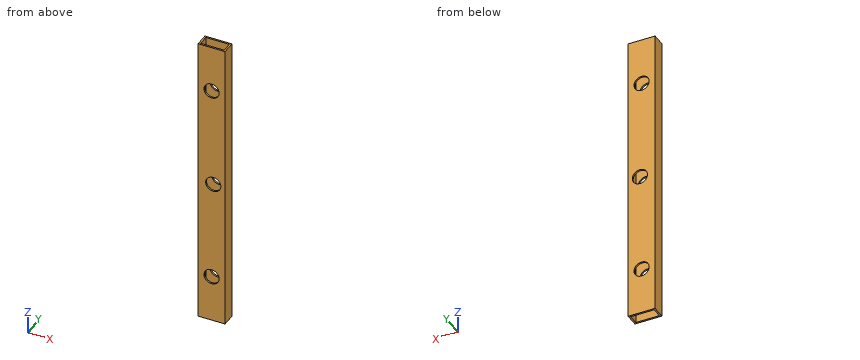
```python
from build123d import *

# Parameters (mm, degrees)
SKETCH1_W           = 50.8
SKETCH1_H           = 25.4
SKETCH1_W_2         = 44.45
SKETCH1_H_2         = 19.05
BOSS_EXTRUDE1_DEPTH = 558.8
SKETCH2_R           = 14.2875
CUT_EXTRUDE1_DEPTH  = 562.678947442


with BuildPart() as part:
    # Sketch1 → Boss-Extrude1 (new body)
    with BuildSketch(Plane.XY):
        with Locations((25.4, 12.7)):
            Rectangle(SKETCH1_W, SKETCH1_H)
        with Locations((25.4, 12.7)):
            Rectangle(SKETCH1_W_2, SKETCH1_H_2, mode=Mode.SUBTRACT)
    extrude(amount=BOSS_EXTRUDE1_DEPTH)

    # Sketch2 → Cut-Extrude1 (cut, through all)
    with BuildSketch(Plane(origin=(0, 25.4, 0), x_dir=(1, 0, 0), z_dir=(0, 1, 0))):
        with Locations(Location((28.575, -279.4, 0), (0, 0, 270))):
            Circle(SKETCH2_R)
        with Locations(Location((25.4, -469.9, 0), (0, 0, 270))):
            Circle(SKETCH2_R)
        with Locations(Location((25.4, -88.9, 0), (0, 0, 90))):
            Circle(SKETCH2_R)
    extrude(amount=-CUT_EXTRUDE1_DEPTH, mode=Mode.SUBTRACT)


solid = part.part
```
CAD build for the part. Positions are in the model's coordinates, mm. Round coordinates to 2 decimals unless told otherwise and drop trailing zeros. Order: outer loops, then holes, each group sorted by start corner. A loop starts at its lowest first (then second) coordinate and runs counter-clockwise, first axis right, second up. Notation, with made-up numbers: (16, 21.25) - (54, 21.25) arc R21 ccw to (54, 30.25) - close; hole circle Ø7 at (23.25, 60.25). An arc over 180 degrees is marked (long way). Answer in a Markdown table with one row per item. Add a question column.
(1) Band-saw the part on A-A on y = 11.5. List the corners of the cut face in (x, z) (3 decimals), and give its area (3 significant figures).
(2) Probe L1, parallel to X at y = 18.5, z = 27 (3 decimals); L2, parallel to Y at x = 37.5, z = 161.5 (3 decimals); L3, parallel to X at y = 23.85, z = 88.9. List the from-to ranges inside material, lowest first. Write a range as [from, to].
(3) Band-saw the part on B-B on z = 434. List the corners of the cut face in (x, y) (3 decimals), and give its area (3 significant figures).
(4) Band-saw the part on C-C on x = 34. Count the separate pieces of the cut face and the enclosed holes in it, and give its area (3 significant figures).
(5) Band-saw the part on D-D on z = 88.9. List the corners of the cut face in (x, y) (1 decimal).
Data:
| question | item | result |
|---|---|---|
| 1 | outline | (0, 0) - (3.175, 0) - (3.175, 558.8) - (0, 558.8) - close; (47.625, 0) - (50.8, 0) - (50.8, 558.8) - (47.625, 558.8) - close |
| 1 | area | 3,550 mm^2 |
| 2 | L1 | x = [0, 3.175], [47.625, 50.8] |
| 2 | L2 | y = [0, 3.175], [22.225, 25.4] |
| 2 | L3 | x = [0, 11.11], [39.69, 50.8] |
| 3 | outline | (0, 0) - (50.8, 0) - (50.8, 25.4) - (0, 25.4) - close; hole (3.175, 3.175) - (47.625, 3.175) - (47.625, 22.225) - (3.175, 22.225) - close |
| 3 | area | 444 mm^2 |
| 4 | separate pieces | 8 |
| 4 | enclosed holes | 0 |
| 4 | area | 3,090 mm^2 |
| 5 | outline | (0, 0) - (11.1, 0) - (11.1, 3.2) - (3.2, 3.2) - (3.2, 22.2) - (11.1, 22.2) - (11.1, 25.4) - (0, 25.4) - close; (39.7, 0) - (50.8, 0) - (50.8, 25.4) - (39.7, 25.4) - (39.7, 22.2) - (47.6, 22.2) - (47.6, 3.2) - (39.7, 3.2) - close |
